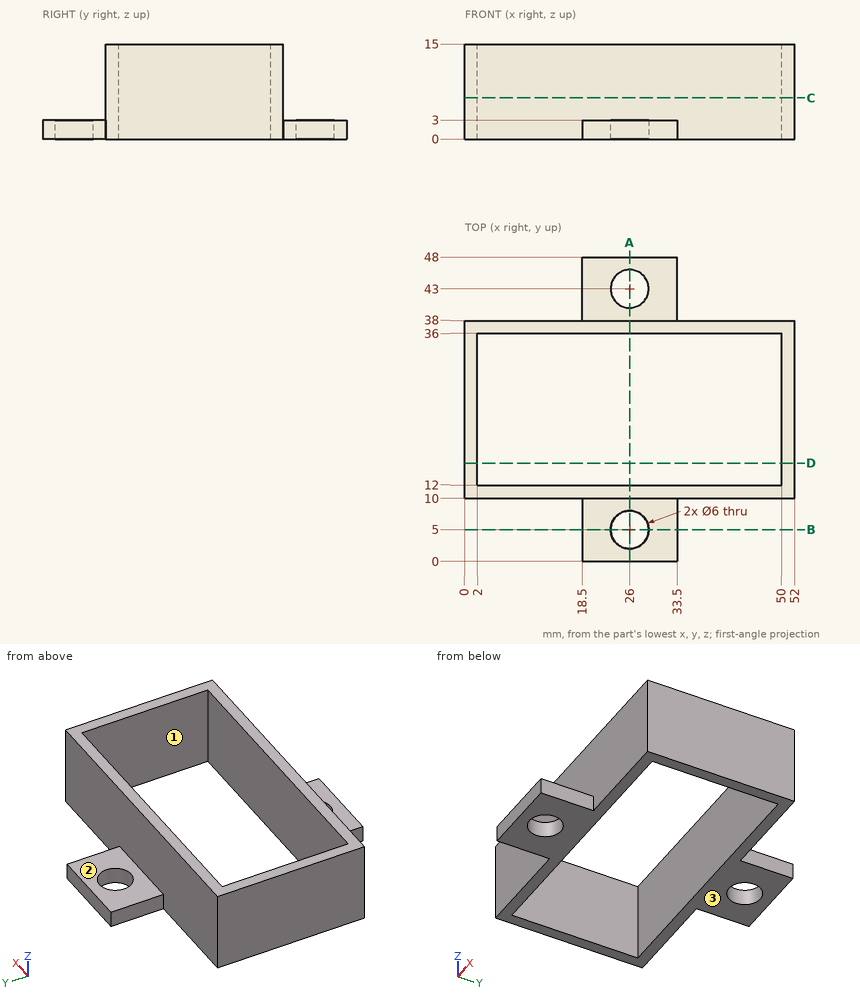
Can you work these out from the drawing? Everything is in mm from the part's minimum corner. A direction names the side the tool comes from. Coordinates: 2 decimals unless noted, no trailing zeros. Order: outer loops, then holes, each group sorted by start corner. A loop starts at its lowest first (then second) coordinate and runs counter-clockwise, first axis right, second up. Notation, with made-up numbers: M -29.5,-23 L 25.5,-23 A34 ccw 25.5,10 Z; hole C 29.25,24.5 d10. An arc over 180 degrees is marked long. Answer as CSV lines item,"result". Start each with the question number.
1. I want a section at C-C, the plane z = 6.5. Write out the boundary of the cut face in (x, y), and give its area (3 significant figures).
2. I want a section at B-B, the plane y = 5. Write out the boundary of the cut face in (x, z), and give its area (3 significant figures).
3. On a 3-axis mill with a long thin cutter (end or side, diameter ignored), from which of +Z, -Z, +X, -X, +Y, -Y can I reach the whole of each face in a straight line? I mean the marked faces 1, 2 and 3. Say none if no direction works.
4. For pin 1 (7.5 mm diameter, centred on x = 29, z = 8, fed in from -Y); pin 2 (2.5 mm diameter, centred on y = 2.5, z = 2, fed in from -X); pin 3 (1 mm diameter, centred on x = 24.5, y = 39.5, fed in from +Z), each with a flat end and sliding along its axis, tell me the tip position at first contact or that it passes through.
5. I want a section at D-D, the plane y = 15.5. Write out the boundary of the cut face in (x, z).
6. I want a section at A-A, the plane x = 26. Write out the boundary of the cut face in (y, z).
7. I need wall thicknesses on line 1 (Y direction, x = 26, z = 1.95); line 2 (Y direction, x = 33.5, z = 9.5); line 3 (X direction, y = 5, z = 1.85). Which ranges of each line are inside material? Lowest first, please. Write a range as [from, to].
Recorded:
1,outline,"M 0,10 L 52,10 L 52,38 L 0,38 Z; hole M 2,12 L 50,12 L 50,36 L 2,36 Z"
1,area,"304 mm2"
2,outline,"M 18.5,0 L 23,0 L 23,3 L 18.5,3 Z; M 29,0 L 33.5,0 L 33.5,3 L 29,3 Z"
2,area,"27.0 mm2"
3,face 1,"+Z, -Z"
3,face 2,"+Z, +X, -X, +Y"
3,face 3,"-Z, +X, -X, +Y, -Y"
4,pin 1,"stops at y = 10"
4,pin 2,"stops at x = 18.5"
4,pin 3,"stops at z = 3"
5,outline,"M 0,0 L 2,0 L 2,15 L 0,15 Z; M 50,0 L 52,0 L 52,15 L 50,15 Z"
6,outline,"M 0,0 L 2,0 L 2,3 L 0,3 Z; M 8,0 L 12,0 L 12,15 L 10,15 L 10,3 L 8,3 Z; M 36,0 L 40,0 L 40,3 L 38,3 L 38,15 L 36,15 Z; M 46,0 L 48,0 L 48,3 L 46,3 Z"
7,line 1,"y = [0, 2], [8, 12], [36, 40], [46, 48]"
7,line 2,"y = [10, 12], [36, 38]"
7,line 3,"x = [18.5, 23], [29, 33.5]"
